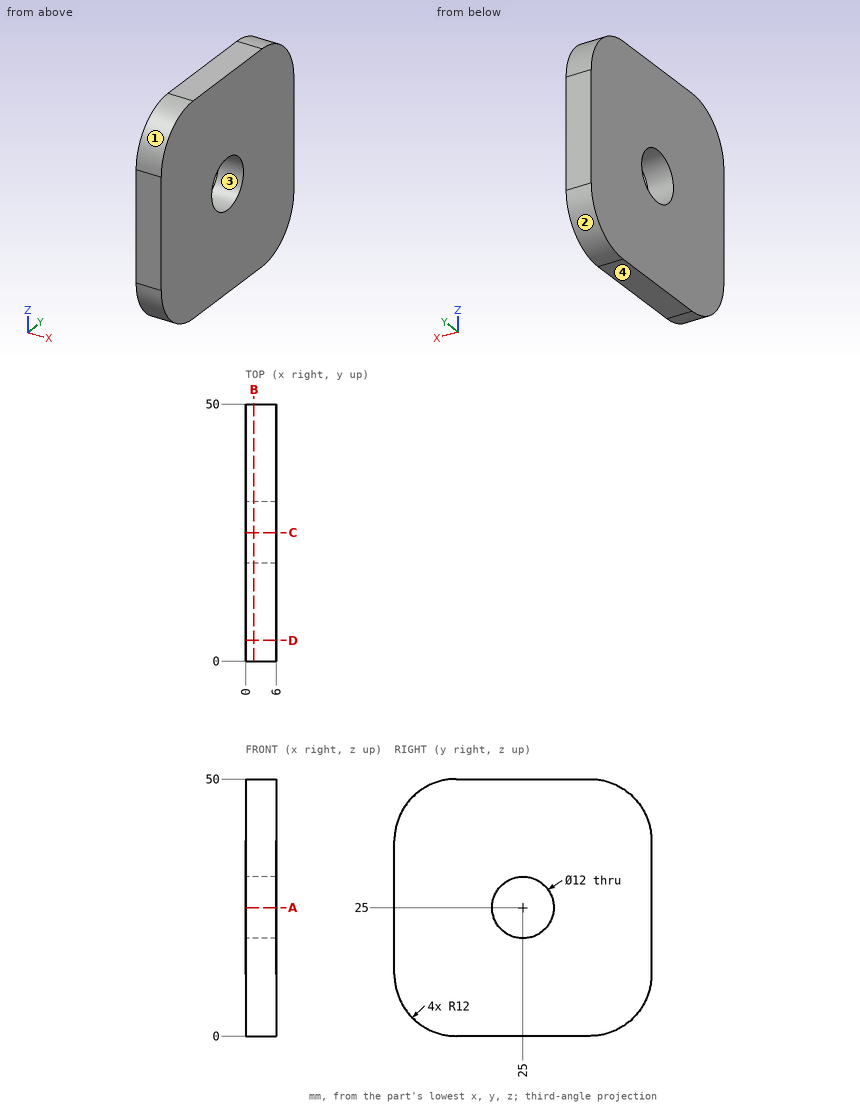
Geometry check sheet. Reference: drawing and pictorial views, mm from the part's lowest x, y, z. Round coordinates to 2 decimals unless told otherwise and drop trailing zeros. Write each loop counter-clockwise with the first axis right and the second up, starting at its lowest first coordinate (ties: lowest second). Pieces come first, ordered by that corner, then holes.
(1) Depth check by flat-ended pin: pin 1 Ø8 at (y, z) = (32, 31) entering from -X; pin 2 Ø11 at (y, z) = (25, 25) entering from -X. Enter the tip coordinate at first touch or a pass-through.
Returned:
pin 1: stops at x = 0
pin 2: passes through
(2) Mould release check, pull along Y, two halves, no side actions. Record for the marked faces 1, 2, 3 and 4: pulls with the +Y half, pulls with the -Y half, needs draft (parallel to the pull), parting line crosses it, or undercut.
Returned:
face 1: pulls with the -Y half
face 2: pulls with the +Y half
face 3: undercut
face 4: needs draft
(3) Section check B-B (x = 1.6). Enter the section's corners in (y, z).
Returned:
outline: (0, 12) arc R12 ccw to (12, 0) - (38, 0) arc R12 ccw to (50, 12) - (50, 38) arc R12 ccw to (38, 50) - (12, 50) arc R12 ccw to (0, 38) - close; hole circle Ø12 at (25, 25)
(4) Material ranges on line 1 (Y direction, x = 4.05, z = 25); line 2 (Y direction, x = 3.4, z = 24), recorded low to high.
Returned:
line 1: y = 0 to 19, 31 to 50
line 2: y = 0 to 19.08, 30.92 to 50
(5) Section check A-A (z = 25). Enter the section's corners in (x, y).
Returned:
outline: (0, 0) - (6, 0) - (6, 19) - (0, 19) - close; (0, 31) - (6, 31) - (6, 50) - (0, 50) - close
(6) Section check D-D (y = 4). Enter the section's corners in (x, z).
Returned:
outline: (0, 3.06) - (6, 3.06) - (6, 46.94) - (0, 46.94) - close
